from build123d import *

# Parameters (mm, degrees)
SKETCH1_W           = 118
SKETCH1_H           = 118
SKETCH1_R           = 2
BOSS_EXTRUDE1_DEPTH = 10
FILLET1_R           = 20


with BuildPart() as part:
    # Sketch1 → Boss-Extrude1 (new body)
    with BuildSketch(Plane(origin=(0, 0, 0), x_dir=(1, 0, 0), z_dir=(0, 1, 0))):
        with Locations((-1.371006445, 1.121732546)):
            Rectangle(SKETCH1_W, SKETCH1_H)
        with Locations(Location((-1.371006445, -46.878267454, 0), (0, 0, 270))):
            Circle(SKETCH1_R, mode=Mode.SUBTRACT)
        with Locations(Location((9.628993555, -46.878267454, 0), (0, 0, 270))):
            Circle(SKETCH1_R, mode=Mode.SUBTRACT)
        with Locations(Location((31.628993555, -46.878267454, 0), (0, 0, 270))):
            Circle(SKETCH1_R, mode=Mode.SUBTRACT)
        with Locations(Location((-34.371006445, -46.878267454, 0), (0, 0, 90))):
            Circle(SKETCH1_R, mode=Mode.SUBTRACT)
        with Locations(Location((-12.371006445, -46.878267454, 0), (0, 0, 90))):
            Circle(SKETCH1_R, mode=Mode.SUBTRACT)
        with Locations(Location((-1.371006445, -9.878267454, 0), (0, 0, 270))):
            Circle(SKETCH1_R, mode=Mode.SUBTRACT)
        with Locations(Location((9.628993555, -9.878267454, 0), (0, 0, 270))):
            Circle(SKETCH1_R, mode=Mode.SUBTRACT)
        with Locations(Location((-12.371006445, -9.878267454, 0), (0, 0, 90))):
            Circle(SKETCH1_R, mode=Mode.SUBTRACT)
        with Locations(Location((-12.371006445, 1.121732546, 0), (0, 0, 270))):
            Circle(SKETCH1_R, mode=Mode.SUBTRACT)
        with Locations(Location((-12.371006445, 12.121732546, 0), (0, 0, 270))):
            Circle(SKETCH1_R, mode=Mode.SUBTRACT)
        with Locations(Location((9.628993555, 12.121732546, 0), (0, 0, 90))):
            Circle(SKETCH1_R, mode=Mode.SUBTRACT)
        with Locations(Location((-1.371006445, 12.121732546, 0), (0, 0, 90))):
            Circle(SKETCH1_R, mode=Mode.SUBTRACT)
        with Locations(Location((-12.371006445, 49.121732546, 0), (0, 0, 270))):
            Circle(SKETCH1_R, mode=Mode.SUBTRACT)
        with Locations(Location((-34.371006445, 49.121732546, 0), (0, 0, 270))):
            Circle(SKETCH1_R, mode=Mode.SUBTRACT)
        with Locations(Location((31.628993555, 49.121732546, 0), (0, 0, 90))):
            Circle(SKETCH1_R, mode=Mode.SUBTRACT)
        with Locations(Location((9.628993555, 49.121732546, 0), (0, 0, 90))):
            Circle(SKETCH1_R, mode=Mode.SUBTRACT)
        with Locations(Location((-1.371006445, 49.121732546, 0), (0, 0, 90))):
            Circle(SKETCH1_R, mode=Mode.SUBTRACT)
        with Locations(Location((9.628993555, 1.121732546, 0), (0, 0, 90))):
            Circle(SKETCH1_R, mode=Mode.SUBTRACT)
        with Locations(Location((46.628993555, 12.121732546, 0), (0, 0, 270))):
            Circle(SKETCH1_R, mode=Mode.SUBTRACT)
        with Locations(Location((46.628993555, 34.121732546, 0), (0, 0, 270))):
            Circle(SKETCH1_R, mode=Mode.SUBTRACT)
        with Locations(Location((46.628993555, -31.878267454, 0), (0, 0, 90))):
            Circle(SKETCH1_R, mode=Mode.SUBTRACT)
        with Locations(Location((46.628993555, -9.878267454, 0), (0, 0, 90))):
            Circle(SKETCH1_R, mode=Mode.SUBTRACT)
        with Locations(Location((46.628993555, 1.121732546, 0), (0, 0, 90))):
            Circle(SKETCH1_R, mode=Mode.SUBTRACT)
        with Locations(Location((-49.371006445, 1.121732546, 0), (0, 0, 270))):
            Circle(SKETCH1_R, mode=Mode.SUBTRACT)
        with Locations(Location((-49.371006445, -9.878267454, 0), (0, 0, 270))):
            Circle(SKETCH1_R, mode=Mode.SUBTRACT)
        with Locations(Location((-49.371006445, -31.878267454, 0), (0, 0, 270))):
            Circle(SKETCH1_R, mode=Mode.SUBTRACT)
        with Locations(Location((-49.371006445, 34.121732546, 0), (0, 0, 90))):
            Circle(SKETCH1_R, mode=Mode.SUBTRACT)
        with Locations(Location((-49.371006445, 12.121732546, 0), (0, 0, 90))):
            Circle(SKETCH1_R, mode=Mode.SUBTRACT)
    extrude(amount=BOSS_EXTRUDE1_DEPTH)

    # Fillet1
    fillet1_edges = [part.edges().sort_by_distance(p)[0] for p in [
        (-60.371006445, 5, -60.121732546),
        (57.628993555, 5, -60.121732546),
        (57.628993555, 5, 57.878267454),
        (-60.371006445, 5, 57.878267454),
    ]]
    fillet(fillet1_edges, radius=FILLET1_R)


solid = part.part
Could you check a few things on this model? Use its own coordinates, in mm. Coordinates: 2 decimals unless noted, no trailing zeros.
1. We'd pull the mould along Z, two halves only. Please class faces 1 (the face through (7.677, 4.93, 9.445)), 2 (the face through (-2, 10, -2)), 3 (the face through (-47.388, 4.93, 31.618)), 4 (the face through (51.615, 5.07, -54.419)): released by +Z, released by -Z, zero draft, split by the parting line, or undercut.
2. I need wall thicknesses on L1, parallel to X at y = 3.25, z = -1; L2, parallel to X at y = 0.5, z = -12.5; L3, parallel to X at y = 7, z = -35. Which ranges of each line are inside material? Lowest first, please.
3. Imagine slicing it at A-A (y = 6.25). Give the number of separate pieces and of enclosed holes in the cut face, and give its area (3 significant figures).
Computed values:
1. face 1: undercut
1. face 2: zero draft
1. face 3: undercut
1. face 4: released by -Z
2. L1: x = -60.37 to -51.37, -47.37 to -14.37, -10.37 to 7.63, 11.63 to 44.63, 48.63 to 57.63
2. L2: x = -60.37 to -51.33, -47.41 to -14.33, -10.41 to -3.33, 0.59 to 7.67, 11.59 to 44.67, 48.59 to 57.63
2. L3: x = -60.37 to -51.17, -47.57 to 44.83, 48.43 to 57.63
3. separate pieces: 1
3. enclosed holes: 28
3. area: 13,200 mm2
